Can you work these out from the model? Positions are in its coordinate system, mm. Face numbers are marked on the shaded views. A direction names the side the tool comes from. Round coordinates to 2 decimals unless told otherwise and drop trailing zeros. Write each loop counter-clockwise with the first axis right and the second up, starting at its lowest first coordinate (ties: lowest second). Pieces come first, ordered by that corner, then holes. Notation, with made-up numbers: M 27,45 L 53,45 A14 ccw 53,62 Z; hole C 57,72 d2. An arc over 180 degrees is marked long. Answer in a Markdown table with one row per item. Add a question column.
(1) I'm going to push flat-ended pins straight in: pin 1 (3 mm diameter, centred on y = 8.5, z = 2, fed in from +X); pin 2 (1.5 mm diameter, centred on y = 0.5, z = 0.5, fed in from +X); pin 3 (2 mm diameter, centred on y = -9.5, z = 7.5, fed in from +X); pin 4 (3 mm diameter, centred on x = 3, y = 9, fed in from +Z). Where does each tip first touch, or does it pass through?
(2) Suppose I cut it at C-C, the plane z = -14. Write out the boundary of the cut face in (x, y), then the cut area to 3 significant figures.
(3) For the marked faces 4, 5 and 6, which set-ups out of +Z, -Z, +X, -X, +Y, -Y let a thin tool reach every point of the face, with its end or its side?
(4) Suppose I cut it at B-B, the plane x = 6. Write out the boundary of the cut face in (y, z), then the cut area to 3 significant figures.
(5) If I drill on probe 1 along Z at (x, y) = (5.3, 0); probe 2 along Y at (x, z) = (1.5, -4); probe 3 along Y at (x, z) = (3, 6), over which ranges is the centre line in solid material (lowest first)?
(6) Suppose I cut it at A-A, the plane x = 3.5. Write out the boundary of the cut face in (y, z), then the cut area to 3 significant figures.
(7) If we mould it in two halves opening along Z, with no side actions, what happens to the marked faces 1, 2 and 3? For each: released by +Z, released by -Z, zero draft, split by the parting line, or undercut.
(8) Suppose I cut it at D-D, the plane y = -15. Write out the boundary of the cut face in (x, z), then the cut area to 3 significant figures.
from build123d import *

# Parameters (mm, degrees)
F0_R      = 17.5
F1_DEPTH  = 5
F3_DEPTH  = 25
F4_R      = 13.5
F5_DEPTH  = 2.5
F6_R      = 1.9999
F7_R      = 1.99
F8_R      = 6
F9_DEPTH  = 0.5
F10_R     = 2.5
F11_DEPTH = 4
F12_R     = 1.5
F13_DEPTH = 4.6


# Not quite as in the source:
# - a fillet or chamfer is up to 0.001 mm smaller than in the source, because OpenCascade refuses the exact size


with BuildPart() as f1:
    # F0 (on Right) → F1 (new body)
    with BuildSketch(Plane.YZ):
        Circle(F0_R)
    extrude(amount=F1_DEPTH)

    # F2 (on face) → F3 (cut)
    with BuildSketch(Plane.YZ.offset(5)):
        with BuildLine():
            Line((-2, 5.6568542495), (-2, 13.3510299228))
            ThreePointArc((-2, 13.3510299228), (-7.9351009059, 10.9217294241), (-12.0795500186, 6.0278081711))
            Line((-12.0795500186, 6.0278081711), (-4.761954107, 3.6501771304))
            ThreePointArc((-4.761954107, 3.6501771304), (-3.5267115138, 4.8541019662), (-2, 5.6568542495))
        make_face()
        with BuildLine():
            Line((4.6626960874, 3.7761442234), (12.1273810063, 5.9309889503))
            ThreePointArc((12.1273810063, 5.9309889503), (7.9787201688, 10.8899047042), (2, 13.3510299228))
            Line((2, 13.3510299228), (2, 5.6568542495))
            ThreePointArc((2, 5.6568542495), (3.4615238464, 4.9008012264), (4.6626960874, 3.7761442234))
        make_face()
        with BuildLine():
            ThreePointArc((9.4655724803, -9.6256395954), (12.4506069829, -5.2184658433), (13.5, 0))
            ThreePointArc((13.5, 0), (13.4581864786, 1.0617046234), (13.3330049322, 2.1168324159))
            Line((13.3330049322, 2.1168324159), (6, 0))
            ThreePointArc((6, 0), (5.7296726323, -1.7806884981), (4.943049491, -3.400920718))
            Line((4.943049491, -3.400920718), (7.7712408853, -7.2935922208))
            Line((7.7712408853, -7.2935922208), (9.4655724803, -9.6256395954))
        make_face()
        with BuildLine():
            ThreePointArc((-6.2295045028, -11.9767806046), (0, -13.5), (6.2295045028, -11.9767806046))
            Line((6.2295045028, -11.9767806046), (4.5351729078, -9.64473323))
            Line((4.5351729078, -9.64473323), (1.7069815135, -5.7520617271))
            ThreePointArc((1.7069815135, -5.7520617271), (0, -6), (-1.7069815135, -5.7520617271))
            Line((-1.7069815135, -5.7520617271), (-6.2295045028, -11.9767806046))
        make_face()
        with BuildLine():
            Line((-9.4655724803, -9.6256395954), (-4.943049491, -3.400920718))
            ThreePointArc((-4.943049491, -3.400920718), (-5.7063390978, -1.8541019662), (-5.9980220845, -0.1540489348))
            Line((-5.9980220845, -0.1540489348), (-13.3156179961, 2.223582106))
            ThreePointArc((-13.3156179961, 2.223582106), (-12.83926297, -4.1717294241), (-9.4655724803, -9.6256395954))
        make_face()
    extrude(amount=-F3_DEPTH, mode=Mode.SUBTRACT)

    # F4 (on face) → F5 (cut)
    with BuildSketch(Plane.YZ.offset(5)):
        Circle(F4_R)
    extrude(amount=-F5_DEPTH, mode=Mode.SUBTRACT)

    # F6 (radius 2 in the source; OpenCascade refuses exactly that, so slightly less here)
    f6_edges = [f1.edges().sort_by_distance(p)[0] for p in [
        (0, -9.65682, 1.034767),
        (0, -8.420752, 4.838993),
        (0, -7.204311, -6.51328),
        (0, -3.968243, -8.864421),
        (0, 3.968243, -8.864421),
        (0, 7.204311, -6.51328),
        (0, 9.666502, 1.058416),
        (0, 2, 9.503942),
        (0, -2, 9.503942),
    ]]
    fillet(f6_edges, radius=F6_R)

    # F7
    f7_edges = [f1.edges().sort_by_distance(p)[0] for p in [
        (0, 8.395039, 4.853567),
    ]]
    fillet(f7_edges, radius=F7_R)

    # F8 (on face) → F9 (join)
    with BuildSketch(Plane.YZ.offset(2.5)):
        Circle(F8_R)
    extrude(amount=F9_DEPTH)

    # F10 (on face) → F11 (join)
    with BuildSketch(Plane.YZ.offset(3)):
        Circle(F10_R)
    extrude(amount=F11_DEPTH)

    # F12 (on face) → F13 (cut)
    with BuildSketch(Plane.YZ.offset(7)):
        Circle(F12_R)
    extrude(amount=-F13_DEPTH, mode=Mode.SUBTRACT)


solid = f1.part
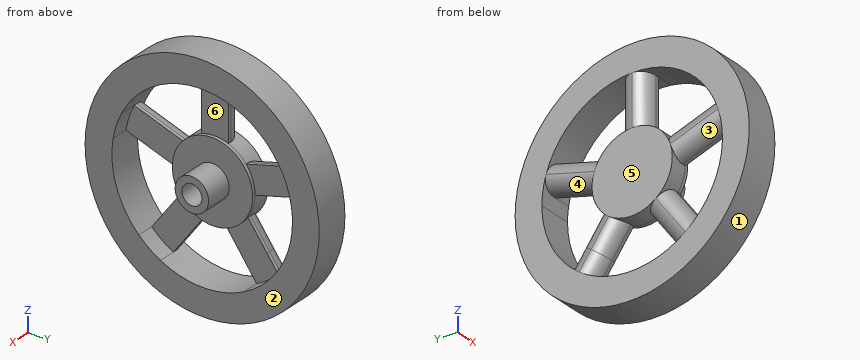
Calculated:
| question | item | result |
|---|---|---|
| 1 | pin 1 | x = 2.5 |
| 1 | pin 2 | x = 2.4 |
| 1 | pin 3 | through |
| 1 | pin 4 | z = 15.81 |
| 2 | outline | M 0,-10.5 L 5,-10.5 L 5,10.5 L 0,10.5 Z |
| 2 | area | 105 mm² |
| 3 | face 4 | -X |
| 3 | face 5 | +Z, -Z, -X, +Y, -Y |
| 3 | face 6 | +X |
| 4 | outline | C 0,0 d5; hole C 0,0 d3 |
| 4 | area | 12.6 mm² |
| 5 | probe 1 | -2.5 to -1.5, 1.5 to 2.5 |
| 5 | probe 2 | -17.04 to -12.89, -5.3 to 5.3, 12.89 to 17.04 |
| 5 | probe 3 | -16.44 to -12.09, 12.09 to 16.44 |
| 6 | outline | C 0,0 d35; C 0,0 d5; hole C 0,0 d27; hole C 0,0 d3 |
| 6 | area | 402 mm² |
| 7 | face 1 | split by the parting line |
| 7 | face 2 | zero draft |
| 7 | face 3 | undercut |
| 8 | outline | M 0,-9.01 L 5,-9.01 L 5,9.01 L 0,9.01 Z |
| 8 | area | 90.1 mm² |
